from build123d import *

# Parameters (mm, degrees)
SKETCH1_W           = 53.3
SKETCH1_H           = 25
BOSS_EXTRUDE1_DEPTH = 11.4
FILLET1_R           = 1
SKETCH2_R           = 3.065
BOSS_EXTRUDE2_DEPTH = 6.1


with BuildPart() as part:
    # Sketch1 → Boss-Extrude1 (new body)
    with BuildSketch(Plane(origin=(0, 0, 0), x_dir=(1, 0, 0), z_dir=(0, 1, 0))):
        Rectangle(SKETCH1_W, SKETCH1_H)
    extrude(amount=BOSS_EXTRUDE1_DEPTH)

    # Fillet1
    fillet1_edges = [part.edges().sort_by_distance(p)[0] for p in [
        (-26.65, 11.4, 0),
        (0, 11.4, 12.5),
        (26.65, 11.4, 0),
        (0, 0, 12.5),
        (-26.65, 0, 0),
        (0, 0, -12.5),
        (26.65, 0, 0),
        (26.65, 5.7, 12.5),
        (-26.65, 5.7, 12.5),
        (-26.65, 5.7, -12.5),
        (26.65, 5.7, -12.5),
        (0, 11.4, -12.5),
    ]]
    fillet(fillet1_edges, radius=FILLET1_R)

    # Sketch2 → Boss-Extrude2 (add)
    with BuildSketch(Plane.ZY.offset(26.65)):
        with Locations((4.975, 6.865)):
            Circle(SKETCH2_R)
    extrude(amount=BOSS_EXTRUDE2_DEPTH)


solid = part.part
Source: CAD feature listing. Evaluate the final solid. Frame: model axes, mm. A direction names the side the tool comes from. Coordinates: 2 decimals unless noted, no trailing zeros. Order: outer loops, then holes, each group sorted by start corner. A loop starts at its lowest first (then second) coordinate and runs counter-clockwise, first axis right, second up. Notation, with made-up numbers: M 7,43.25 L 56,43.25 A20 ccw 56,52.25 Z; hole C 28.25,47.25 d3. An arc over 180 degrees is marked long. Write each question's results on one line, items separated by ' | '. Start each with the question number.
1. Reachability of faces 1 (the face through (-29.657, 3.873, 4.311)), 2 (the face through (0.359, 0.301, 12.215)) from +Z, -Z, +X, -X, +Y, -Y: full face, straight path, thin tool, end or side. Return the list, or none.
2. Section A-A, the plane y = 5.25. Return the cut outline in (x, z).
3. Material intervals for L1, parallel to X at y = 5.75, z = 2; L2, parallel to Z at x = 15.5, y = 10.5; L3, parallel to Z at x = -2, y = 0.5, sorted ascending.
4. Section C-C, the plane y = 9.25. Return the cut outline in (x, z).
5. Section B-B, the plane z = -8.75. Return the cut outline in (x, y).
Solution:
1) face 1: -X | face 2: +Z, +X, -X, -Y
2) outline: M -32.75,2.37 L -26.65,2.37 L -26.65,-11.5 A1 ccw -25.65,-12.5 L 25.65,-12.5 A1 ccw 26.65,-11.5 L 26.65,11.5 A1 ccw 25.65,12.5 L -25.65,12.5 A1 ccw -26.65,11.5 L -26.65,7.58 L -32.75,7.58 Z
3) L1: -26.65 to 26.65 | L2: -12.49 to 12.49 | L3: -12.37 to 12.37
4) outline: M -32.75,3.05 L -26.65,3.05 L -26.65,-11.5 A1 ccw -25.65,-12.5 L 25.65,-12.5 A1 ccw 26.65,-11.5 L 26.65,11.5 A1 ccw 25.65,12.5 L -25.65,12.5 A1 ccw -26.65,11.5 L -26.65,6.9 L -32.75,6.9 Z
5) outline: M -26.65,1 A1 ccw -25.65,0 L 25.65,0 A1 ccw 26.65,1 L 26.65,10.4 A1 ccw 25.65,11.4 L -25.65,11.4 A1 ccw -26.65,10.4 Z
